Read the model definition and answer for the solid it produces. Units are mm, in the model's axes. Face numbers are marked on the shaded views. A direction names the side the tool comes from. Give positions to 0.01 mm unless a question says otherwise; leave off trailing zeros. Order: outer loops, then holes, each group sorted by start corner. A loop starts at its lowest first (then second) coordinate and runs counter-clockwise, first axis right, second up.
Item 1: A cutting plane is placed at C-C (z = -297). Write down the section's boundary in (x, y), plus the area to 3 significant figures.
Item 2: Given pin 1 Ø1 at (y, z) = (0.5, -94) entering from +X; pin 2 Ø8 at (x, y) = (28, -27.5) entering from +Z; pin 3 Ø3 at (x, y) = (32, 68.5) entering from -Z, each flat-ended and moving along its own axis, determine where each tip first touches the part or whether it passes through.
Item 3: The mould has two halves that part along Z. Classify the marked faces 1, 2 and 3: +Z half, -Z half, draft (parallel to the pull), parting line (faces both ways), or undercut.
Item 4: Which of the six approach directions +Z, -Z, +X, -X, +Y, -Y give full straight-line access (tool end or side, diameter ignored) to the marked faces 4, 5 and 6?
Item 5: A cutting plane is placed at B-B (y = 0). Write down the section's boundary in (x, z), plus the area to 3 significant figures.
Item 6: Find the intervals of material crossed by line 1 along Z through (x, y) = (-26.5, -60.5); line 2 along X through (y, z) = (5, -260); line 3 along X through (y, z) = (48, 5), in increasing order.
Item 7: A cutting plane is placed at A-A (x = 0). Write down the section's boundary in (y, z).
from build123d import *

# Parameters (mm, degrees)
SKETCH1_R           = 100
BOSS_EXTRUDE1_DEPTH = 40
SKETCH2_R           = 15
BOSS_EXTRUDE2_DEPTH = 20
SKETCH3_R           = 20
BOSS_EXTRUDE3_DEPTH = 495
CUT_EXTRUDE1_START  = -250
SKETCH4_OUTSIDE_W   = 326.584
SKETCH4_OUTSIDE_H   = 326.584
SKETCH4_OUTSIDE_R   = 17
CUT_EXTRUDE1_DEPTH  = 50
CHAMFER1_SIZE       = 5
FILLET1_R           = 5
CUT_EXTRUDE2_START  = -104.02
SKETCH5_R           = 20
CUT_EXTRUDE2_DEPTH  = 104.02


with BuildPart() as part:
    # Sketch1 → Boss-Extrude1 (new body)
    with BuildSketch(Plane.XY):
        Circle(SKETCH1_R)
    extrude(amount=BOSS_EXTRUDE1_DEPTH)

    # Sketch2 → Boss-Extrude2 (add)
    with BuildSketch(Plane.XY.offset(40)):
        with Locations((0, 50)):
            Circle(SKETCH2_R)
        with Locations((43.301270189, -25)):
            Circle(SKETCH2_R)
        with Locations((-43.301270189, -25)):
            Circle(SKETCH2_R)
    extrude(amount=BOSS_EXTRUDE2_DEPTH)

    # Sketch3 → Boss-Extrude3 (add)
    with BuildSketch(Plane(origin=(0, 0, 0), x_dir=(-1, 0, 0), z_dir=(0, 0, -1))):
        Circle(SKETCH3_R)
    extrude(amount=BOSS_EXTRUDE3_DEPTH)

    # Sketch4 outside → Cut-Extrude1 (cut)
    with BuildSketch(Plane(origin=(0, 0, -495), x_dir=(-1, 0, 0), z_dir=(0, 0, -1)).offset(CUT_EXTRUDE1_START)):
        Rectangle(SKETCH4_OUTSIDE_W, SKETCH4_OUTSIDE_H)
        Circle(SKETCH4_OUTSIDE_R, mode=Mode.SUBTRACT)
    extrude(amount=-CUT_EXTRUDE1_DEPTH, mode=Mode.SUBTRACT)

    # Chamfer1
    chamfer1_edges = [part.edges().sort_by_distance(p)[0] for p in [
        (-58.301270189, -25, 60),
        (-15, 50, 60),
        (28.301270189, -25, 60),
    ]]
    chamfer(chamfer1_edges, length=CHAMFER1_SIZE)

    # Fillet1
    fillet1_edges = [part.edges().sort_by_distance(p)[0] for p in [
        (-100, 0, 40),
    ]]
    fillet(fillet1_edges, radius=FILLET1_R)

    # Sketch5 → Cut-Extrude2 (cut)
    with BuildSketch(Plane(origin=(0, 0, -495), x_dir=(-1, 0, 0), z_dir=(0, 0, -1)).offset(CUT_EXTRUDE2_START)):
        Circle(SKETCH5_R)
    extrude(amount=CUT_EXTRUDE2_DEPTH, mode=Mode.SUBTRACT)


solid = part.part
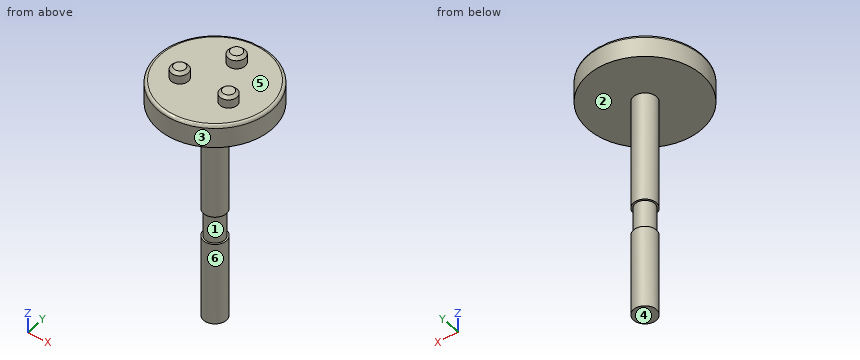
Response values:
1. outline: circle Ø40 at (0, 0)
1. area: 1,260 mm2
2. pin 1: stops at x = 20
2. pin 2: stops at z = 58.5
2. pin 3: stops at z = 0
3. face 1: undercut
3. face 2: -Z half
3. face 3: draft
4. face 4: -Z, +X, -X, +Y, -Y
4. face 5: +Z
4. face 6: -Z
5. outline: (-100, 0) - (-20, 0) - (-20, -195) - (-17, -195) - (-17, -245) - (-20, -245) - (-20, -390.98) - (20, -390.98) - (20, -245) - (17, -245) - (17, -195) - (20, -195) - (20, 0) - (100, 0) - (100, 35) arc R5 ccw to (95, 40) - (-95, 40) arc R5 ccw to (-100, 35) - close
5. area: 23,300 mm2
6. line 1: z = 0 to 40
6. line 2: x = -19.36 to 19.36
6. line 3: x = -87.73 to 87.73
7. outline: (-100, 0) - (-20, 0) - (-20, -195) - (-17, -195) - (-17, -245) - (-20, -245) - (-20, -390.98) - (20, -390.98) - (20, -245) - (17, -245) - (17, -195) - (20, -195) - (20, 0) - (100, 0) - (100, 35) arc R5 ccw to (95, 40) - (65, 40) - (65, 55) - (60, 60) - (40, 60) - (35, 55) - (35, 40) - (-95, 40) arc R5 ccw to (-100, 35) - close
